Read the model definition and answer for the solid it produces. Units are mm, in the model's axes. A direction names the side the tool comes from. Give positions to 0.01 mm unless a question says otherwise; leave off trailing zeros. Order: outer loops, then holes, each group sorted by start corner. A loop starts at its lowest first (then second) coordinate and runs counter-clockwise, first axis right, second up. Notation, with made-up numbers: (-9.5, 68) -> (14.5, 68) arc R17 cw to (14.5, 84) -> close; hole circle Ø8 at (73.5, -28). An arc over 180 degrees is marked (long way). Answer as CSV lines item,"result". Start each with the question number.
1) The mould has two halves that part along Z. Classify faces 1 (the face through (66.82, 11.79, -0.52)), 2 (the face through (96.65, 3, 9)), 3 (the face through (23.353, -12.204, 4.859)): +Z half, -Z half, draft (parallel to the pull), parting line (faces both ways), or undercut.
2) Find section C-C (x = 74). Determine the outline of the cut face in (y, z).
3) For faces 4 (the face through (36.15, -9, 9)), 5 (the face through (-55.42, 11.79, -0.52)), 6 (the face through (-23.291, -12.487, -4.797)), 7 (the face through (-74.15, 3, 9)), determine the directions among +Z, -Z, +X, -X, +Y, -Y from which every point of the face is accessible in a straight line to the end or side of a thin tool.
4) Straight lines are drawn through the part: L1, parallel to X at y = -15.5, z = -1.5; L2, parallel to Z at x = -34.4, y = -16.55; L3, parallel to X at y = 14, z = -9. For each, find the intervals that lie inside material, in ascending order. Write a range as from..to.
5) Flat-ended cylindrical pins translate along their axes: pin 1 Ø4 at (y, z) = (-8.28, -14.33) entering from +X; pin 2 Ø1.5 at (y, z) = (8.28, -14.33) entering from -X; pin 3 Ø12 at (x, y) = (-49, 3) entering from +Z; pin 4 Ø5.5 at (y, z) = (-2, 0) entering from +X. Find the tip coordinate at first contact, or state that the pin passes through.
6) Find section B-B (z = 3.5). State how many separate pieces and enclosed holes the cut face has, and give its area (3 significant figures).
7) Find section A-A (x = 4.5). Determine the outline of the cut face in (y, z).
```python
from build123d import *

# Parameters (mm, degrees)
CIRPATTERN1_COUNT   = 6
CUT_EXTRUDE2_START  = 22.15
CUT_EXTRUDE2_DEPTH  = 10
FILLET1_R           = 4
MIRROR1_START       = -36.15
MIRROR1_OUTLINE_R   = 1.25
MIRROR1_DEPTH       = 8.4999999
MIRROR1_START_2     = -28.15
MIRROR1_2_OUTLINE_R = 1.25
MIRROR1_2_DEPTH     = 6
MIRROR1_START_3     = -21
MIRROR1_3_DEPTH     = 21


with BuildPart() as part:
    # Sketch1 → Revolve1 (revolve)
    with BuildSketch(Plane.XY, mode=Mode.PRIVATE) as revolve1_sk:
        Polygon((0, 6), (0, 20.3), (36.15, 20.3), (36.15, 11.8), (96.65, 11.8), (96.65, 9), (88.65, 9), (88.65, 6), align=None)
    revolve(revolve1_sk.sketch.rotate(Axis((-6.306589334, 0, 0), (1, 0, 0)), 180), axis=Axis((-6.306589334, 0, 0), (1, 0, 0)))

    # Sketch4 → M3 Tapped Hole1 (revolve, cut)
    with BuildSketch(Plane(origin=(36.15, 16.55, 0), x_dir=(0, 0, -1), z_dir=(0, 1, 0))):
        Polygon((0, 0), (0, 9.251075774), (1.25, 8.5), (1.25, 0), align=None)
    m3_tapped_hole1 = revolve(axis=Axis((42.5, 16.55, 0), (-1, 0, 0)), mode=Mode.SUBTRACT)

    # CirPattern1: M3 Tapped Hole1 ×6 about axis
    cirpattern1_axis = Axis((0, 0, 0), (1, 0, 0))
    for i in range(1, CIRPATTERN1_COUNT):
        add(m3_tapped_hole1.rotate(cirpattern1_axis, i * 360 / CIRPATTERN1_COUNT), mode=Mode.SUBTRACT)

    # Sketch5 → Cut-Extrude2 (cut)
    with BuildSketch(Plane(origin=(0, 0, 0), x_dir=(0, 0, -1), z_dir=(1, 0, 0)).offset(CUT_EXTRUDE2_START)):
        with BuildLine():
            Line((-6, 0), (-6, -19.393039989))
            ThreePointArc((-6, -19.393039989), (0, -20.3), (6, -19.393039989))
            Line((6, -19.393039989), (6, 0))
            ThreePointArc((6, 0), (0, -6), (-6, 0))
        make_face()
    extrude(amount=CUT_EXTRUDE2_DEPTH, mode=Mode.SUBTRACT)

    # Sketch1<3> → Revolve2 (revolve)
    with BuildSketch(Plane.XY, mode=Mode.PRIVATE) as revolve2_sk:
        Polygon((-66.15, 9), (-66.15, 6), (0, 6), (0, 20.3), (-36.15, 20.3), (-36.15, 11.8), (-74.15, 11.8), (-74.15, 9), align=None)
    revolve(revolve2_sk.sketch.rotate(Axis((-6.306589334, 0, 0), (1, 0, 0)), 180), axis=Axis((-6.306589334, 0, 0), (1, 0, 0)))

    # Fillet1
    # the kernel refuses this fillet: 4 mm, written as the material it adds along each edge
    with BuildSketch(Plane(origin=(32.15, 10, 6), x_dir=(-1, 0, 0), z_dir=(0, -1, 0))) as fillet1_piece_1_section:
        with BuildLine():
            CenterArc((FILLET1_R, FILLET1_R), FILLET1_R, 180, 90)
            Line((0, FILLET1_R), (0, 0))
            Line((0, 0), (FILLET1_R, 0))
        make_face()
    fillet1_piece_1 = extrude(amount=39.393039989, mode=Mode.PRIVATE)
    fillet1_piece_1 = fillet1_piece_1 - Plane(origin=(32.15, 0, 0), x_dir=(0, -1, 0), z_dir=(-1, 0, 0)) * Cylinder(6, 95, mode=Mode.PRIVATE)
    fillet1_piece_1 = fillet1_piece_1 & Plane(origin=(32.15, 0, 0), x_dir=(0, -1, 0), z_dir=(1, 0, 0)) * Cylinder(20.3, 95, mode=Mode.PRIVATE)
    add(fillet1_piece_1)
    with BuildSketch(Plane(origin=(32.15, -29.393039989, -6), x_dir=(-1, 0, 0), z_dir=(0, 1, 0))) as fillet1_piece_2_section:
        with BuildLine():
            CenterArc((FILLET1_R, FILLET1_R), FILLET1_R, 180, 90)
            Line((0, FILLET1_R), (0, 0))
            Line((0, 0), (FILLET1_R, 0))
        make_face()
    fillet1_piece_2 = extrude(amount=39.393039989, mode=Mode.PRIVATE)
    fillet1_piece_2 = fillet1_piece_2 - Plane(origin=(32.15, 0, 0), x_dir=(0, -1, 0), z_dir=(-1, 0, 0)) * Cylinder(6, 95, mode=Mode.PRIVATE)
    fillet1_piece_2 = fillet1_piece_2 & Plane(origin=(32.15, 0, 0), x_dir=(0, -1, 0), z_dir=(1, 0, 0)) * Cylinder(20.3, 95, mode=Mode.PRIVATE)
    add(fillet1_piece_2)
    with BuildSketch(Plane(origin=(22.15, 10, 6), x_dir=(0, 0, -1), z_dir=(0, -1, 0))) as fillet1_piece_3_section:
        with BuildLine():
            CenterArc((FILLET1_R, FILLET1_R), FILLET1_R, 180, 90)
            Line((0, FILLET1_R), (0, 0))
            Line((0, 0), (FILLET1_R, 0))
        make_face()
    fillet1_piece_3 = extrude(amount=39.393039989, mode=Mode.PRIVATE)
    fillet1_piece_3 = fillet1_piece_3 - Plane(origin=(22.15, 0, 0), x_dir=(0, -1, 0), z_dir=(-1, 0, 0)) * Cylinder(6, 95, mode=Mode.PRIVATE)
    fillet1_piece_3 = fillet1_piece_3 & Plane(origin=(22.15, 0, 0), x_dir=(0, -1, 0), z_dir=(1, 0, 0)) * Cylinder(20.3, 95, mode=Mode.PRIVATE)
    add(fillet1_piece_3)
    with BuildSketch(Plane(origin=(22.15, -29.393039989, -6), x_dir=(1, 0, 0), z_dir=(0, 1, 0))) as fillet1_piece_4_section:
        with BuildLine():
            CenterArc((FILLET1_R, -FILLET1_R), FILLET1_R, 90, 90)
            Line((0, -FILLET1_R), (0, 0))
            Line((0, 0), (FILLET1_R, 0))
        make_face()
    fillet1_piece_4 = extrude(amount=39.393039989, mode=Mode.PRIVATE)
    fillet1_piece_4 = fillet1_piece_4 - Plane(origin=(22.15, 0, 0), x_dir=(0, -1, 0), z_dir=(-1, 0, 0)) * Cylinder(6, 95, mode=Mode.PRIVATE)
    fillet1_piece_4 = fillet1_piece_4 & Plane(origin=(22.15, 0, 0), x_dir=(0, -1, 0), z_dir=(1, 0, 0)) * Cylinder(20.3, 95, mode=Mode.PRIVATE)
    add(fillet1_piece_4)

    # Mirror1: read off the stored shape, not the designer's step
    # Mirror1 outline → Mirror1 (cut)
    with BuildSketch(Plane.YZ.offset(MIRROR1_START)):
        with Locations((8.275, -14.332720433)):
            Circle(MIRROR1_OUTLINE_R)
        with Locations((-8.275, -14.332720433)):
            Circle(MIRROR1_OUTLINE_R)
        with Locations((-16.55, 0)):
            Circle(MIRROR1_OUTLINE_R)
        with Locations((-8.275, 14.332720433)):
            Circle(MIRROR1_OUTLINE_R)
        with Locations((8.275, 14.332720433)):
            Circle(MIRROR1_OUTLINE_R)
        with Locations((16.55, 0)):
            Circle(MIRROR1_OUTLINE_R)
    extrude(amount=MIRROR1_DEPTH, mode=Mode.SUBTRACT)

    # Mirror1 2 outline → Mirror1 2 (cut)
    with BuildSketch(Plane.YZ.offset(MIRROR1_START_2)):
        with Locations((-16.55, 0)):
            Circle(MIRROR1_2_OUTLINE_R)
    extrude(amount=MIRROR1_2_DEPTH, mode=Mode.SUBTRACT)

    # Mirror1 3 outline → Mirror1 3 (cut)
    with BuildSketch(Plane(origin=(0, 0, 0), x_dir=(1, 0, 0), z_dir=(0, 1, 0)).offset(MIRROR1_START_3)):
        with BuildLine():
            ThreePointArc((-28.15, 6), (-30.978427125, 4.828427125), (-32.15, 2))
            Line((-32.15, 2), (-32.15, -2))
            ThreePointArc((-32.15, -2), (-30.978427125, -4.828427125), (-28.15, -6))
            Line((-28.15, -6), (-26.15, -6))
            ThreePointArc((-26.15, -6), (-23.321572875, -4.828427125), (-22.15, -2))
            Line((-22.15, -2), (-22.15, 2))
            ThreePointArc((-22.15, 2), (-23.321572875, 4.828427125), (-26.15, 6))
            Line((-26.15, 6), (-28.15, 6))
        make_face()
    extrude(amount=MIRROR1_3_DEPTH, mode=Mode.SUBTRACT)

    # Mirror1 4 outline → Mirror1 4 (revolve, cut)
    with BuildSketch(Plane(origin=(0, 8.275, -14.332720433), x_dir=(0, 1, 0), z_dir=(0, 0, -1))):
        Polygon((1.25, -27.65), (0, -26.898924226), (0, -27.6500001), align=None)
    revolve(axis=Axis((0, 8.275, -14.332720433), (1, 0, 0)), mode=Mode.SUBTRACT)

    # Mirror1 5 outline → Mirror1 5 (revolve, cut)
    with BuildSketch(Plane(origin=(0, -8.275, -14.332720433), x_dir=(0, 1, 0), z_dir=(0, 0, -1))):
        Polygon((1.25, -27.65), (0, -26.898924226), (0, -27.6500001), align=None)
    revolve(axis=Axis((0, -8.275, -14.332720433), (1, 0, 0)), mode=Mode.SUBTRACT)

    # Mirror1 6 outline → Mirror1 6 (revolve, cut)
    with BuildSketch(Plane(origin=(0, -8.275, 14.332720433), x_dir=(0, 1, 0), z_dir=(0, 0, -1))):
        Polygon((1.25, -27.65), (0, -26.898924226), (0, -27.6500001), align=None)
    revolve(axis=Axis((0, -8.275, 14.332720433), (1, 0, 0)), mode=Mode.SUBTRACT)

    # Mirror1 7 outline → Mirror1 7 (revolve, cut)
    with BuildSketch(Plane(origin=(0, 8.275, 14.332720433), x_dir=(0, 1, 0), z_dir=(0, 0, -1))):
        Polygon((1.25, -27.65), (0, -26.898924226), (0, -27.6500001), align=None)
    revolve(axis=Axis((0, 8.275, 14.332720433), (1, 0, 0)), mode=Mode.SUBTRACT)

    # Mirror1 8 outline → Mirror1 8 (revolve, cut)
    with BuildSketch(Plane(origin=(0, 16.55, 0), x_dir=(0, 1, 0), z_dir=(0, 0, -1))):
        Polygon((1.25, -27.65), (0, -26.898924226), (0, -27.6500001), align=None)
    revolve(axis=Axis((0, 16.55, 0), (1, 0, 0)), mode=Mode.SUBTRACT)


solid = part.part
```
Findings below:
1,face 1,"parting line"
1,face 2,"draft"
1,face 3,"undercut"
2,outline,"circle Ø23.6 at (0, 0); hole circle Ø12 at (0, 0)"
3,face 4,"+X"
3,face 5,"-X"
3,face 6,"-Y"
3,face 7,"+Z, -Z, -X, +Y, -Y"
4,L1,"-36.15..-32.15, -22.15..22.15, 32.15..36.15"
4,L2,"-11.76..-1.25, 1.25..11.76"
4,L3,"-36.15..36.15"
5,pin 1,"x = 36.15"
5,pin 2,"x = -27.35"
5,pin 3,"z = 11.8"
5,pin 4,"through"
6,separate pieces,"4"
6,enclosed holes,"0"
6,area,"3,050 mm²"
7,outline,"circle Ø40.6 at (0, 0); hole circle Ø12 at (0, 0)"
